```python
from build123d import *

# Parameters (mm, degrees)
F0_W     = 100
F0_H     = 100
F1_DEPTH = 100
F2_R     = 10
F3_DEPTH = 25
F4_R     = 1.2


with BuildPart() as f1:
    # F0 (on Top) → F1 (new body)
    with BuildSketch(Plane.XY):
        Rectangle(F0_W, F0_H)
    extrude(amount=F1_DEPTH)

    # F2 (on face) → F3 (cut)
    with BuildSketch(Plane.XY.offset(100)):
        Circle(F2_R)
    extrude(amount=-F3_DEPTH, mode=Mode.SUBTRACT)

    # F4
    f4_edges = [f1.edges().sort_by_distance(p)[0] for p in [
        (-50, 0, 100),
        (0, 50, 100),
        (50, 0, 100),
        (0, -50, 100),
        (-50, -50, 50),
        (-50, 50, 50),
        (50, -50, 50),
        (50, 50, 50),
        (50, 0, 0),
        (0, -50, 0),
        (-50, 0, 0),
        (0, 50, 0),
    ]]
    fillet(f4_edges, radius=F4_R)


solid = f1.part
```
Design review of the part built by this model. Coordinates are the model's own, in mm. A direction names the side the tool comes from. Give positions to 0.01 mm unless a question says otherwise; leave off trailing zeros. Order: outer loops, then holes, each group sorted by start corner. A loop starts at its lowest first (then second) coordinate and runs counter-clockwise, first axis right, second up. Notation, with made-up numbers: (39, 79.25) - (43, 79.25) arc R21 ccw to (43, 108.25) - close; hole circle Ø10 at (54.5, 76). An arc over 180 degrees is marked (long way). Use a Markdown table: item, result. Add a question column.
(1) Add section A-A on y = 0. Give the boundary of the cut face in (x, z), then the cut area to 3 significant figures.
(2) Mouldability with a two-part tool opening along X and no side actions: class faces 1 (the face through (-2.17, -9.76, 87.68)), 2 (the face through (-1, 12, 100)), 3 (the face through (-50, -1, 49)) as +X half, -X half, draft (parallel to the pull), parting line (faces both ways), or undercut.
(3) Machinability: for faces 4 (the face through (0, 0, 75)), 5 (the face through (50, -1, 49)), which of the approach directions +Z, -Z, +X, -X, +Y, -Y give a long, thin tool a straight path to every point of the face, cutting with its end or side? Answer none if there is none.
(4) Clearance check with a flat-ended pin moving along its axis: P1, Ø16, axis at x = -2.5, y = -4, coming from the +Z side. State where the tip first meets the part, or that it passes through.
(5) Wall thickness on probe 1 along Y at (x, z) = (0, 83): over which ranges is the line inside the solid? List them lowest first. Write a range as [from, to].
Report:
| question | item | result |
|---|---|---|
| 1 | outline | (-50, 1.2) arc R1.2 ccw to (-48.8, 0) - (48.8, 0) arc R1.2 ccw to (50, 1.2) - (50, 98.8) arc R1.2 ccw to (48.8, 100) - (10, 100) - (10, 75) - (-10, 75) - (-10, 100) - (-48.8, 100) arc R1.2 ccw to (-50, 98.8) - close |
| 1 | area | 9,500 mm² |
| 2 | face 1 | undercut |
| 2 | face 2 | draft |
| 2 | face 3 | -X half |
| 3 | face 4 | +Z |
| 3 | face 5 | +Z, -Z, +X, +Y, -Y |
| 4 | P1 | stops at z = 100 |
| 5 | probe 1 | y = [-50, -10], [10, 50] |
